Geometry check sheet. Reference: drawing and pictorial views, mm from the part's lowest x, y, z. A direction names the side the tool comes from. Give positions to 0.01 mm unless a question says otherwise; leave off trailing zeros. Write each loop counter-clockwise with the first axis right and the second up, starting at its lowest first coordinate (ties: lowest second). Pieces come first, ordered by that corner, then holes. Notation, with made-up numbers: M -16.5,52 L 20.5,52 A16 ccw 20.5,79 Z; hole C -12.75,62.5 d2. An arc over 180 degrees is marked long. Answer as a JSON object with one key per item and string values.
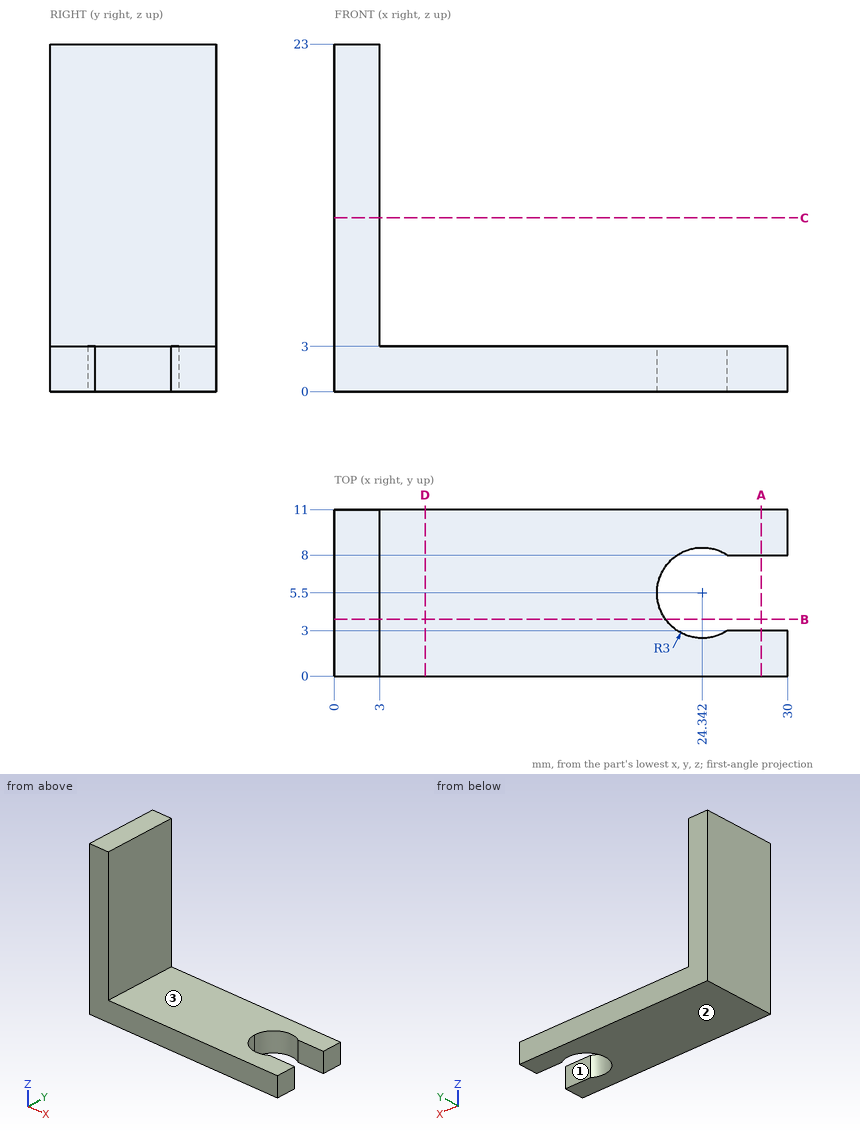
1) Thickness scan on L1, parallel to X at y = 7.5, z = 20. Record the ranges inside material, lowest first.
Completed:
{"L1": "x = 0 to 3"}
2) Section check C-C on z = 11.5. Record the boundary of the cut face in (x, y).
Completed:
{"outline": "M 0,0 L 3,0 L 3,11 L 0,11 Z"}
3) Section check A-A on x = 28.25. Record the boundary of the cut face in (y, z), and give its area (3 significant figures).
Completed:
{"outline": "M 0,0 L 3,0 L 3,3 L 0,3 Z; M 8,0 L 11,0 L 11,3 L 8,3 Z", "area": "18.0 mm2"}
4) Access from +Z, -Z, +X, -X, +Y, -Y to the whole of each face (thin tool, end or side, straight path). Record for the marked faces 1, 2 and 3.
Completed:
{"face 1": "+Z, -Z, +X", "face 2": "-Z, +X, -X, +Y, -Y", "face 3": "+Z, +X, +Y, -Y"}
5) Go/stop test with flat-tipped pins: pin 1 (4 mm diameter, centred on x = 5.5, z = 10, fed in from -Y); pin 2 (4 mm diameter, centred on y = 2, z = 8.5, fed in from +X); pin 3 (1.5 mm diameter, centred on x = 17.5, y = 6, fed in from +Z). Record where each tip stops, or that it passes through.
Completed:
{"pin 1": "passes through", "pin 2": "stops at x = 3", "pin 3": "stops at z = 3"}
6) Section check D-D on x = 6. Record the boundary of the cut face in (y, z), and give its area (3 significant figures).
Completed:
{"outline": "M 0,0 L 11,0 L 11,3 L 0,3 Z", "area": "33.0 mm2"}
7) Section check B-B on y = 3.75. Record the boundary of the cut face in (x, z) (1 decimal), and give its area (3 significant figures).
Completed:
{"outline": "M 0,0 L 21.9,0 L 21.9,3 L 3,3 L 3,23 L 0,23 Z", "area": "126 mm2"}
